Design review of the part built by this model. Coordinates are the model's own, in mm. A direction names the side the tool comes from. Coordinates: 2 decimals unless noted, no trailing zeros. Write each loop counter-clockwise with the first axis right and the second up, starting at its lowest first coordinate (ties: lowest second). Pieces come first, ordered by that corner, then holes. Notation, with made-up numbers: (-38.5, -18.75) -> (-33.5, -18.75) arc R7 cw to (-33.5, -12.75) -> close; hole circle Ø5 at (37.25, -13.5). An arc over 180 degrees is marked (long way). Answer in a Markdown table with one row per item. Add a question column.
Item 1: For faces 4 (the face through (11.853, 1.467, 1.479)), 5 (the face through (9.018, -1, 1)), list the 3-axis set-ups (+Z, -Z, +X, -X, +Y, -Y) from which the entire face can be reached by the end or side of a thin tool; tool diameter is ignored.
Item 2: Take a section at A-A, the plane y = -19. Write out the cut boundary in (x, z).
Item 3: Draft analysis for pull direction Y (two halves, no side actions). For faces 1 (the face through (20, 0, 1)), 2 (the face through (14, 7.332, 1)), 3 (the face through (5.953, -17.843, 1.479)), state which applies: released by +Y, released by -Y, zero draft, split by the parting line, or undercut.
Item 4: Take a section at D-D, the plane x = 8. Write out the cut boundary in (y, z), and give its area (3 significant figures).
Item 5: Take a section at C-C, the plane z = 2.45. Write out the cut boundary in (x, y), and give its area (3 significant figures).
Item 6: To check wall thickness, follow line 1 (X direction, y = 1.5, z = 0.85); line 2 (X direction, y = -4.5, z = 0.2); line 3 (X direction, y = 3, z = 2.4). State the ranges of each line that lie inside material, in increasing order.
Item 7: Take a section at B-B, the plane x = 3.5. Write out the cut boundary in (y, z).
Item 8: Clearance check with a flat-ended pin moving along its axis: P1, Ø1, axis at y = -12, z = 1, coming from the -X side. State where the tip first meets the part, or that it passes through.
from build123d import *

# Parameters (mm, degrees)
SKETCH2_R           = 2
BOSS_EXTRUDE1_DEPTH = 3


with BuildPart() as part:
    # Sketch2 → Boss-Extrude1 (new body)
    with BuildSketch(Plane(origin=(0, 0, 0), x_dir=(-1, 0, 0), z_dir=(0, 0, 1))):
        with BuildLine():
            Line((-9.017950721, -7.332311194), (-20, -7.332311194))
            Line((-20, -7.332311194), (-20, 7.332311194))
            ThreePointArc((-20, 7.332311194), (-12.680293068, 21.732536084), (3.26719031, 24.305930805))
            Line((3.26719031, 24.305930805), (1.482539955, 15.227759845))
            Line((1.482539955, 15.227759845), (-9.017950721, 8.920221357))
            Line((-9.017950721, 8.920221357), (-9.017950721, -7.332311194))
        make_face()
        with Locations(Location((-13.851036571, -1.379219301, 0), (0, 0, 180))):
            Circle(SKETCH2_R, mode=Mode.SUBTRACT)
        with Locations(Location((-4.045326452, 18.443425538, 0), (0, 0, 180))):
            Circle(SKETCH2_R, mode=Mode.SUBTRACT)
    extrude(amount=BOSS_EXTRUDE1_DEPTH)


solid = part.part
Answers:
| question | item | result |
|---|---|---|
| 1 | face 4 | +Z, -Z |
| 1 | face 5 | +Z, -Z, -X, +Y |
| 2 | outline | (-2.22, 0) -> (2.12, 0) -> (2.12, 3) -> (-2.22, 3) -> close; (5.97, 0) -> (15.65, 0) -> (15.65, 3) -> (5.97, 3) -> close |
| 3 | face 1 | zero draft |
| 3 | face 2 | released by +Y |
| 3 | face 3 | undercut |
| 4 | outline | (-24.18, 0) -> (-9.53, 0) -> (-9.53, 3) -> (-24.18, 3) -> close |
| 4 | area | 43.9 mm^2 |
| 5 | outline | (-3.27, -24.31) arc R17.82 ccw to (20, -7.33) -> (20, 7.33) -> (9.02, 7.33) -> (9.02, -8.92) -> (-1.48, -15.23) -> close; hole circle Ø4 at (4.05, -18.44); hole circle Ø4 at (13.85, 1.38) |
| 5 | area | 409 mm^2 |
| 6 | line 1 | x = 9.02 to 11.85, 15.85 to 20 |
| 6 | line 2 | x = 9.02 to 20 |
| 6 | line 3 | x = 9.02 to 12.68, 15.02 to 20 |
| 7 | outline | (-25.11, 0) -> (-20.37, 0) -> (-20.37, 3) -> (-25.11, 3) -> close; (-16.52, 0) -> (-12.23, 0) -> (-12.23, 3) -> (-16.52, 3) -> close |
| 8 | P1 | stops at x = 3.06 |
